Read the model definition and answer for the solid it produces. Units are mm, in the model's axes. Face numbers are marked on the shaded views. A direction names the side the tool comes from. Give positions to 0.01 mm unless a question says otherwise; leave off trailing zeros. Loops run counter-clockwise (first coordinate to the right, second up) from the corner with the lowest first, then second, coordinate; pieces in that order, holes last. Notation, with made-up numbers: (52, 88.25) -> (67, 88.25) arc R34 ccw to (67, 124.25) -> close; hole circle Ø9 at (4.5, -6.75). An arc over 180 degrees is marked (long way). Return JSON: item names as keys, results as strings. Group by question number.
from build123d import *

# Parameters (mm, degrees)
BOSS_EXTRUDE1_DEPTH = 2
BOSS_EXTRUDE2_DEPTH = 8
SKETCH24_R          = 3.9
BOSS_EXTRUDE5_DEPTH = 4.4
SKETCH30_W          = 4.40861202
SKETCH30_H          = 1.324178481
CUT_EXTRUDE12_DEPTH = 16
CUT_EXTRUDE11_DEPTH = 23.928148639
FILLET1_R           = 1.5
SKETCH34_W          = 1.5
SKETCH34_H          = 1.5
CUT_EXTRUDE13_DEPTH = 8
SKETCH36_R          = 0.95
CUT_EXTRUDE15_DEPTH = 8
SKETCH37_R          = 2
CUT_EXTRUDE16_DEPTH = 4.5
SKETCH38_W          = 3
SKETCH38_H          = 1.25
CUT_EXTRUDE17_DEPTH = 3.6


with BuildPart() as part:
    # Sketch2 → Boss-Extrude1 (new body)
    with BuildSketch(Plane.XY):
        with BuildLine():
            Line((-2.5, 7.5), (-16.7, 7.5))
            Line((-16.7, 7.5), (-20.7, 3.793442666))
            Line((-20.7, 3.793442666), (-20.7, -4.031648778))
            Line((-20.7, -4.031648778), (-15.7, -7.5))
            Line((-15.7, -7.5), (-6.7, -7.5))
            Line((-6.7, -7.5), (-4.2, -5.6))
            ThreePointArc((-4.2, -5.6), (3.130495168, -6.260990337), (7, 0))
            ThreePointArc((7, 0), (4.949747468, 4.949747468), (0, 7))
            Line((0, 7), (0, 7.5))
            Line((0, 7.5), (-2.5, 7.5))
        make_face()
    extrude(amount=BOSS_EXTRUDE1_DEPTH)

    # Sketch4 → Boss-Extrude2 (add)
    with BuildSketch(Plane.XY.offset(2)):
        Polygon((-15.7, -7.5), (-6.7, -7.5), (-6.759079174, -4.5), (-7.7, -4.5), (-7.7, 2), (-5.5, 2), (-5.5, 5.3), (-2.5, 5.3), (-2.5, 7.5), (-16.7, 7.5), (-20.7, 3.793442666), (-20.7, -4.031648778), align=None)
    extrude(amount=BOSS_EXTRUDE2_DEPTH)

    # Sketch24 → Boss-Extrude5 (add)
    with BuildSketch(Plane.XY.offset(2)):
        Circle(SKETCH24_R)
    extrude(amount=BOSS_EXTRUDE5_DEPTH)

    # Sketch30 → Cut-Extrude12 (cut)
    with BuildSketch(Plane(origin=(-5.5, 0, 0), x_dir=(0, 0, -1), z_dir=(1, 0, 0))):
        with Locations((-4.20430601, 4.63791076)):
            Rectangle(SKETCH30_W, SKETCH30_H)
    extrude(amount=-CUT_EXTRUDE12_DEPTH, mode=Mode.SUBTRACT)

    # Sketch28 → Cut-Extrude11 (cut, through all)
    with BuildSketch(Plane.XY.offset(6.4)):
        with BuildLine():
            Line((-1, 0.979795897), (-1, -0.979795897))
            ThreePointArc((-1, -0.979795897), (1.4, 0), (-1, 0.979795897))
        make_face()
    extrude(amount=-CUT_EXTRUDE11_DEPTH, mode=Mode.SUBTRACT)

    # Fillet1
    # the kernel refuses this fillet: 1.5 mm, written as the material it takes off along each edge
    with BuildSketch(Plane(origin=(-15.230677435, -6, 1.5), x_dir=(-0.5699665637840448, -0.8216678867816415, 0), z_dir=(0, 0, -1))) as fillet1_piece_1_section:
        Polygon((0, 0), (FILLET1_R * 1.02, 0), (FILLET1_R * 1.02, -FILLET1_R * 0.319139344377), (FILLET1_R * 0.838101244517, -FILLET1_R * 0.58136589506), align=None)
    fillet1_piece_1 = extrude(amount=FILLET1_R * 1.02, mode=Mode.PRIVATE)
    fillet1_piece_1 = fillet1_piece_1 - Plane(origin=(-15.230677435, -6, 1.5), x_dir=(0.29860685961507855, 0.9543762064253388, 0), z_dir=(0, 0, -1)) * Sphere(FILLET1_R, mode=Mode.PRIVATE)
    add(fillet1_piece_1, mode=Mode.SUBTRACT)
    with BuildSketch(Plane(origin=(-16.11186344, 6, 1.5), x_dir=(-0.6796897201843015, 0.7334997506991983, 0), z_dir=(0, 0, -1))) as fillet1_piece_2_section:
        Polygon((0, 0), (FILLET1_R * 1.02, 0), (FILLET1_R * 1.02, FILLET1_R * 0.399932860855), (FILLET1_R * 0.748169745713, FILLET1_R * 0.693283514588), align=None)
    fillet1_piece_2 = extrude(amount=FILLET1_R * 1.02, mode=Mode.PRIVATE)
    fillet1_piece_2 = fillet1_piece_2 - Plane(origin=(-16.11186344, 6, 1.5), x_dir=(0.3650344157067945, -0.9309940254102596, 0), z_dir=(0, 0, -1)) * Sphere(FILLET1_R, mode=Mode.PRIVATE)
    add(fillet1_piece_2, mode=Mode.SUBTRACT)
    with BuildSketch(Plane(origin=(-19.2, 3.138411196, 1.5), x_dir=(-0.6796897201843015, 0.7334997506991983, 0), z_dir=(0, 0, -1))) as fillet1_piece_3_section:
        Polygon((0, 0), (FILLET1_R * 1.02, 0), (FILLET1_R * 1.02, -FILLET1_R * 0.445421399395), (FILLET1_R * 0.693283514588, -FILLET1_R * 0.748169745713), align=None)
    fillet1_piece_3 = extrude(amount=FILLET1_R * 1.02, mode=Mode.PRIVATE)
    fillet1_piece_3 = fillet1_piece_3 - Plane(origin=(-19.2, 3.138411196, 1.5), x_dir=(0.9164304993244992, -0.40019387789901173, 0), z_dir=(0, 0, -1)) * Sphere(FILLET1_R, mode=Mode.PRIVATE)
    add(fillet1_piece_3, mode=Mode.SUBTRACT)
    with BuildSketch(Plane(origin=(-19.2, -3.246599046, 1.5), x_dir=(-0.5699665637840448, -0.8216678867816415, 0), z_dir=(0, 0, -1))) as fillet1_piece_4_section:
        Polygon((0, 0), (FILLET1_R * 1.02, 0), (FILLET1_R * 1.02, FILLET1_R * 0.533833817771), (FILLET1_R * 0.58136589506, FILLET1_R * 0.838101244517), align=None)
    fillet1_piece_4 = extrude(amount=FILLET1_R * 1.02, mode=Mode.PRIVATE)
    fillet1_piece_4 = fillet1_piece_4 - Plane(origin=(-19.2, -3.246599046, 1.5), x_dir=(0.8859928227090906, 0.46369895202380795, 0), z_dir=(0, 0, -1)) * Sphere(FILLET1_R, mode=Mode.PRIVATE)
    add(fillet1_piece_4, mode=Mode.SUBTRACT)
    with BuildSketch(Plane(origin=(-15.230677435, -7.5, 0), x_dir=(0, 1, 0), z_dir=(1, 0, 0))) as fillet1_piece_5_section:
        with BuildLine():
            CenterArc((FILLET1_R, FILLET1_R), FILLET1_R, 180, 90)
            Line((0, FILLET1_R), (0, 0))
            Line((0, 0), (FILLET1_R, 0))
        make_face()
    fillet1_piece_5 = extrude(amount=12.280677435, mode=Mode.PRIVATE)
    fillet1_piece_5 = split(fillet1_piece_5, bisect_by=Plane(origin=(-9.092127217, -9.318016685, 0.3282266), z_dir=(-0.6050832675335577, 0.7961621941231027, 0)), keep=Keep.TOP, mode=Mode.PRIVATE)
    add(fillet1_piece_5, mode=Mode.SUBTRACT)
    with BuildSketch(Plane(origin=(3.75, 7.5, 0), x_dir=(0, 0, 1), z_dir=(-1, 0, 0))) as fillet1_piece_6:
        with BuildLine():
            CenterArc((FILLET1_R, -FILLET1_R), FILLET1_R, 90, 90)
            Line((0, -FILLET1_R), (0, 0))
            Line((0, 0), (FILLET1_R, 0))
        make_face()
    extrude(amount=19.86186344, mode=Mode.SUBTRACT)
    with BuildSketch(Plane(origin=(-17.13139802, 7.100249626, 0), x_dir=(0.6796897201843014, -0.7334997506991981, 0), z_dir=(-0.7334997506991983, -0.6796897201843015, 0))) as fillet1_piece_7:
        with BuildLine():
            CenterArc((FILLET1_R, FILLET1_R), FILLET1_R, 180, 90)
            Line((0, FILLET1_R), (0, 0))
            Line((0, 0), (FILLET1_R, 0))
        make_face()
    extrude(amount=4.21013989, mode=Mode.SUBTRACT)
    with BuildSketch(Plane(origin=(-20.054949846, -4.479100876, 0), x_dir=(0.5699665637840448, 0.8216678867816416, 0), z_dir=(0.8216678867816415, -0.5699665637840448, 0))) as fillet1_piece_8:
        with BuildLine():
            CenterArc((FILLET1_R, FILLET1_R), FILLET1_R, 180, 90)
            Line((0, FILLET1_R), (0, 0))
            Line((0, 0), (FILLET1_R, 0))
        make_face()
    extrude(amount=4.830811364, mode=Mode.SUBTRACT)
    with BuildSketch(Plane(origin=(-20.7, 3.138411196, 0), x_dir=(1, 0, 0), z_dir=(0, -1, 0))) as fillet1_piece_9:
        with BuildLine():
            CenterArc((FILLET1_R, FILLET1_R), FILLET1_R, 180, 90)
            Line((0, FILLET1_R), (0, 0))
            Line((0, 0), (FILLET1_R, 0))
        make_face()
    extrude(amount=6.385010242, mode=Mode.SUBTRACT)
    with BuildSketch(Plane(origin=(-15.7, -7.5, 1.5), x_dir=(1, 0, 0), z_dir=(0, 0, 1))) as fillet1_piece_10:
        with BuildLine():
            CenterArc((FILLET1_R * 0.312881710173, FILLET1_R), FILLET1_R, 235.252105822, 34.747894178)
            Line((-FILLET1_R * 0.257084853611, FILLET1_R * 0.178332113218), (0, 0))
            Line((0, 0), (FILLET1_R * 0.312881710173, 0))
        make_face()
    extrude(amount=9.673306413, mode=Mode.SUBTRACT)
    with BuildSketch(Plane(origin=(-20.7, -4.031648778, 1.5), x_dir=(0, 1, 0), z_dir=(0, 0, 1))) as fillet1_piece_11:
        with BuildLine():
            CenterArc((FILLET1_R * 0.523366488011, -FILLET1_R), FILLET1_R, 90, 55.252105822)
            Line((-FILLET1_R * 0.298301398771, -FILLET1_R * 0.430033436216), (0, 0))
            Line((0, 0), (FILLET1_R * 0.523366488011, 0))
        make_face()
    extrude(amount=10.46262433, mode=Mode.SUBTRACT)
    with BuildSketch(Plane(origin=(-20.7, 3.793442666, 1.5), x_dir=(0.7334997506991984, 0.6796897201843014, 0), z_dir=(0, 0, 1))) as fillet1_piece_12:
        with BuildLine():
            CenterArc((FILLET1_R * 0.436687646465, -FILLET1_R), FILLET1_R, 90, 47.18059856)
            Line((-FILLET1_R * 0.296812104234, -FILLET1_R * 0.320310279816), (0, 0))
            Line((0, 0), (FILLET1_R * 0.436687646465, 0))
        make_face()
    extrude(amount=10.137578674, mode=Mode.SUBTRACT)
    with BuildSketch(Plane(origin=(-16.7, 7.5, 1.5), x_dir=(1, 0, 0), z_dir=(0, 0, 1))) as fillet1_piece_13:
        with BuildLine():
            CenterArc((FILLET1_R * 0.392091040054, -FILLET1_R), FILLET1_R, 90, 42.81940144)
            Line((-FILLET1_R * 0.287598680131, -FILLET1_R * 0.266500249301), (0, 0))
            Line((0, 0), (FILLET1_R * 0.392091040054, 0))
        make_face()
    extrude(amount=9.9703414, mode=Mode.SUBTRACT)

    # Sketch34 → Cut-Extrude13 (cut, along a direction that is not the sketch's normal)
    with BuildSketch(Plane.XZ.offset(-2)):
        with Locations((-6.95, 10)):
            Rectangle(SKETCH34_W, SKETCH34_H)
    extrude(amount=-CUT_EXTRUDE13_DEPTH, dir=(0.6685833876565112, -0.7436371788377336, 0), mode=Mode.SUBTRACT)

    # Sketch36 → Cut-Extrude15 (cut)
    with BuildSketch(Plane.XY.offset(10)):
        with Locations((-11.7, 0)):
            Circle(SKETCH36_R)
        with Locations((-16.7, 0)):
            Circle(SKETCH36_R)
    extrude(amount=-CUT_EXTRUDE15_DEPTH, mode=Mode.SUBTRACT)

    # Sketch37 → Cut-Extrude16 (cut)
    with BuildSketch(Plane(origin=(0, 0, 0), x_dir=(-1, 0, 0), z_dir=(0, 0, -1))):
        with Locations((11.7, 0)):
            Circle(SKETCH37_R)
        with Locations((16.7, 0)):
            Circle(SKETCH37_R)
    extrude(amount=-CUT_EXTRUDE16_DEPTH, mode=Mode.SUBTRACT)

    # Sketch38 → Cut-Extrude17 (cut)
    with BuildSketch(Plane.XY.offset(10)):
        with Locations((-4, 5.925)):
            Rectangle(SKETCH38_W, SKETCH38_H)
    extrude(amount=-CUT_EXTRUDE17_DEPTH, mode=Mode.SUBTRACT)


solid = part.part
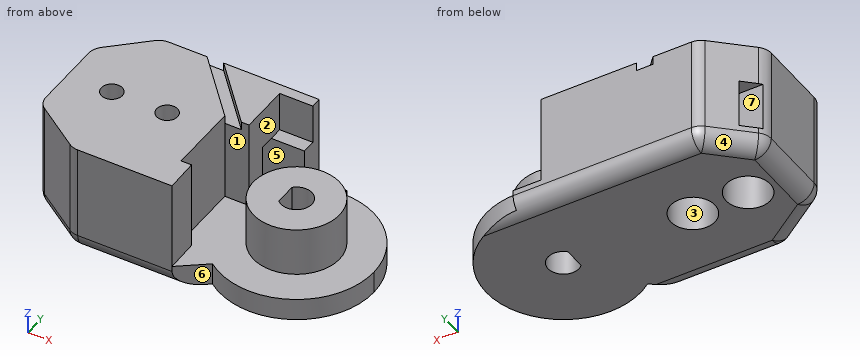
1. Which of the six approach directions +Z, -Z, +X, -X, +Y, -Y give full straight-line access (tool end or side, diameter ignored) to the marked faces 1, 2 and 3?
2. Section D-D on x = 1 is taken. Determine the outline of the cut face in (y, z), then the cut area to 3 significant figures.
3. Section C-C on z = 7 is taken. Determine the outline of the cut face in (x, y), then the cut area to 3 significant figures.
4. Flat-ended cylindrical pins translate along their axes: pin 1 Ø0.6 at (x, y) = (-3.5, 5.5) entering from +Z; pin 2 Ø1.7 at (x, y) = (-16.7, 0) entering from -Z; pin 3 Ø1.4 at (y, z) = (3.5, 7.5) entering from +X. Find the tip coordinate at first contact, or state that the pin passes through.
5. Section A-A on z = 3.75 is taken. Determine the outline of the cut face in (x, y), then the cut area to 3 significant figures.
6. Straight lines are drawn through the part: line 1 (Y direction, x = -7.25, z = 3.25); line 2 (Y direction, x = 0, z = 2.5); line 3 (Y direction, x = -13.25, z = 6.25). For each, find the intervals that lie inside material, in ascending order. Write a range as from..to.
7. Section B-B on x = -11.7 is taken. Determine the outline of the cut face in (y, z).
8. Determine the mould class of the marked faces 4, 5, 6 and 7 for opening direction Z: pulls with the +Z half, pulls with the -Z half, needs draft (parallel to the pull), parting line crosses it, or undercut.
Completed:
{
 "1": {"face 1": "+Z", "face 2": "+Z, -Y", "face 3": "-Z"},
 "2": {"outline": "(-6.93, 0) -> (-0.98, 0) -> (-0.98, 6.4) -> (-3.77, 6.4) -> (-3.77, 2) -> (-6.93, 2) -> close; (0.98, 0) -> (6, 0) arc R1.5 ccw to (6.93, 0.32) -> (6.93, 2) -> (3.77, 2) -> (3.77, 6.4) -> (0.98, 6.4) -> close", "area": "48.2 mm²"},
 "3": {"outline": "(-20.7, -3.25) arc R1.5 ccw to (-20.05, -4.48) -> (-16.09, -7.23) arc R1.5 ccw to (-15.23, -7.5) -> (-6.7, -7.5) -> (-6.76, -4.5) -> (-7.7, -4.5) -> (-7.7, 2) -> (-5.5, 2) -> (-5.5, 6.55) -> (-2.5, 6.55) -> (-2.5, 7.5) -> (-16.11, 7.5) arc R1.5 ccw to (-17.13, 7.1) -> (-20.22, 4.24) arc R1.5 ccw to (-20.7, 3.14) -> close; hole circle Ø1.9 at (-16.7, 0); hole circle Ø1.9 at (-11.7, 0)", "area": "191 mm²"},
 "4": {"pin 1": "stops at z = 6.4", "pin 2": "passes through", "pin 3": "stops at x = -5.5"},
 "5": {"outline": "(-20.7, -3.25) arc R1.5 ccw to (-20.05, -4.48) -> (-16.09, -7.23) arc R1.5 ccw to (-15.23, -7.5) -> (-6.7, -7.5) -> (-6.76, -4.5) -> (-7.7, -4.5) -> (-7.7, 2) -> (-5.5, 2) -> (-5.5, 3.98) -> (-20.44, 3.98) arc R1.5 ccw to (-20.7, 3.14) -> close; (-19.07, 5.3) -> (-2.5, 5.3) -> (-2.5, 7.5) -> (-16.11, 7.5) arc R1.5 ccw to (-17.13, 7.1) -> close; circle Ø7.8 at (0, 0); hole circle Ø4 at (-16.7, 0); hole circle Ø4 at (-11.7, 0); hole (-1, -0.98) arc R1.4 ccw (long way) to (-1, 0.98) -> close", "area": "198 mm²"},
 "6": {"line 1": "y = -7.5..-4.5, 2..3.98, 5.3..7.5", "line 2": "y = -3.9..-1.4, 1.4..3.9", "line 3": "y = -7.5..3.98, 5.3..7.5"},
 "7": {"outline": "(-7.5, 1.5) arc R1.5 ccw to (-6, 0) -> (-2, 0) -> (-2, 4.5) -> (-0.95, 4.5) -> (-0.95, 10) -> (-7.5, 10) -> close; (0.95, 4.5) -> (2, 4.5) -> (2, 0) -> (6, 0) arc R1.5 ccw to (7.5, 1.5) -> (7.5, 9.25) -> (6.45, 9.25) -> (6.45, 10) -> (0.95, 10) -> close; hole (3.98, 2) -> (5.3, 2) -> (5.3, 6.41) -> (3.98, 6.41) -> close"},
 "8": {"face 4": "pulls with the -Z half", "face 5": "undercut", "face 6": "needs draft", "face 7": "undercut"}
}
